Autodesk Inventor part; units mm, degrees
ref_plane "YZ Plane" through (0, 0, 0) normal (1, 0, 0) x (0, 1, 0)
ref_plane "XZ Plane" through (0, 0, 0) normal (0, 1, 0) x (-1, 0, 0)
ref_plane "XY Plane" through (0, 0, 0) normal (0, 0, 1) x (1, 0, 0)
sketch "Sketch1" plane through (0, 0, 0) normal (1, 0, 0) x (0, 1, 0)
  circle A0 centre (0, 0) radius 10
  circle A1 centre (0, 0) radius 20.6375
  line L0 (0, 0) -> (0, 44)
  circle A2 centre (0, 44) radius 2.5
  line L1 (20.6375, 0) -> (-20.6375, 0)
  arc A3 (6, 44) -> (-6, 44) centre (0, 44) ccw
  line L2 (6, 44) -> (6, 29.3939)
  line L3 (-6, 44) -> (-6, 29.3939)
  circle A4 centre (0, -44) radius 2.5
  arc A5 (-6, -44) -> (6, -44) centre (0, -44) ccw
  line L4 (6, -44) -> (6, -29.3939)
  line L5 (-6, -44) -> (-6, -29.3939)
  arc A6 (-6, 29.3939) -> (-6, -29.3939) centre (0, 0) ccw
  arc A7 (6, -29.3939) -> (6, 29.3939) centre (0, 0) ccw
  dimension "d0" = 20
  dimension "d1" = 41.275
  dimension "d5" = 44
  dimension "d6" = 5
  dimension "d7" = 12
extrude "Extrusion1" add sketch "Sketch1" along normal blind 5
properties part number "Sujetador_Rodamiento"
Geometry check sheet. Reference: the model listing, model coordinates, mm. A direction names the side the tool comes from. Give positions to 0.01 mm unless a question says otherwise; leave off trailing zeros. Write each loop counter-clockwise with the first axis right and the second up, starting at its lowest first coordinate (ties: lowest second). Pieces come first, ordered by that corner, then holes. Notation, with made-up numbers: M 88,65 L 104,65 A26 ccw 104,96 Z; hole C 1.5,13 d5. An arc over 180 degrees is marked long. Answer as CSV lines item,"result". Start each with the question number.
Q1. Section check C-C, the plane x = 4.15. Record the cut outline in (y, z) (1 decimal), then the cut area to 3 significant figures.
Q2. Section check D-D, the plane z = -37. Record the cut outline in (x, y), then the cut area to 3 significant figures.
Q3. Go/stop test with flat-tipped pins: pin 1 (1 mm diameter, centred on y = 12, z = -14.5, fed in from -X); pin 2 (2.5 mm diameter, centred on x = 2, z = -33.5, fed in from +Y); pin 3 (3 mm diameter, centred on x = 1.5, z = 11.5, fed in from +Y). Record where each tip stops, or that it passes through.
Q4. Tool access check on faces 1 (the face through (2, 6, -37)), 2 (the face through (2, -6, 37)), 3 (the face through (2.465, -29.995, -0.575)), 4 (the face through (2, -6, -37)). Record the directions out of +Z, -Z, +X, -X, +Y, -Y that give a thin tool (end or side, any length) a straight path to the whole face; none if there is none.
Q5. Material ranges on L1, parallel to Z at x = 3.2, y = 0; L2, parallel to Y at x = 3.05, z = 44; L3, parallel to Z at x = 4.2, y = 1.5, recorded low to high.
Q6. Section check A-A, the plane z = 0. Record the cut outline in (x, y), then the cut area to 3 significant figures.
Q7. Release check for a two-part mould opening along Y. For faces 5 (the face through (2, 0, 50)), 6 (the face through (2.46, -0.54, 46.44)), 7 (the face through (2, 6, 37)) record: pulls with the +Y half, pulls with the -Y half, needs draft (parallel to the pull), parting line crosses it, or undercut.
Q8. Section check B-B, the plane y = 0. Record the cut outline in (x, z), then the cut area to 3 significant figures.
Geometry says:
1,outline,"M -6,-44 A6 ccw 6,-44 L 6,-29.4 A30 ccw 6,29.4 L 6,44 A6 ccw -6,44 L -6,29.4 A30 ccw -6,-29.4 Z; hole C 0,0 d41.3; hole C 0,-44 d5; hole C 0,44 d5"
1,area,"1,900 mm^2"
2,outline,"M 0,-6 L 5,-6 L 5,6 L 0,6 Z"
2,area,"60.0 mm^2"
3,pin 1,"through"
3,pin 2,"y = 6"
3,pin 3,"y = 28.28"
4,face 1,"-Z, +X, -X, +Y"
4,face 2,"+Z, +X, -X, -Y"
4,face 3,"+X, -X, -Y"
4,face 4,"-Z, +X, -X, -Y"
5,L1,"-50 to -46.5, -41.5 to -20.64, 20.64 to 41.5, 46.5 to 50"
5,L2,"-6 to -2.5, 2.5 to 6"
5,L3,"-49.81 to -46, -42 to -20.58, 20.58 to 42, 46 to 49.81"
6,outline,"M 0,-30 L 5,-30 L 5,-20.64 L 0,-20.64 Z; M 0,20.64 L 5,20.64 L 5,30 L 0,30 Z"
6,area,"93.6 mm^2"
7,face 5,"parting line crosses it"
7,face 6,"undercut"
7,face 7,"pulls with the +Y half"
8,outline,"M 0,-50 L 5,-50 L 5,-46.5 L 0,-46.5 Z; M 0,-41.5 L 5,-41.5 L 5,-20.64 L 0,-20.64 Z; M 0,20.64 L 5,20.64 L 5,41.5 L 0,41.5 Z; M 0,46.5 L 5,46.5 L 5,50 L 0,50 Z"
8,area,"244 mm^2"
